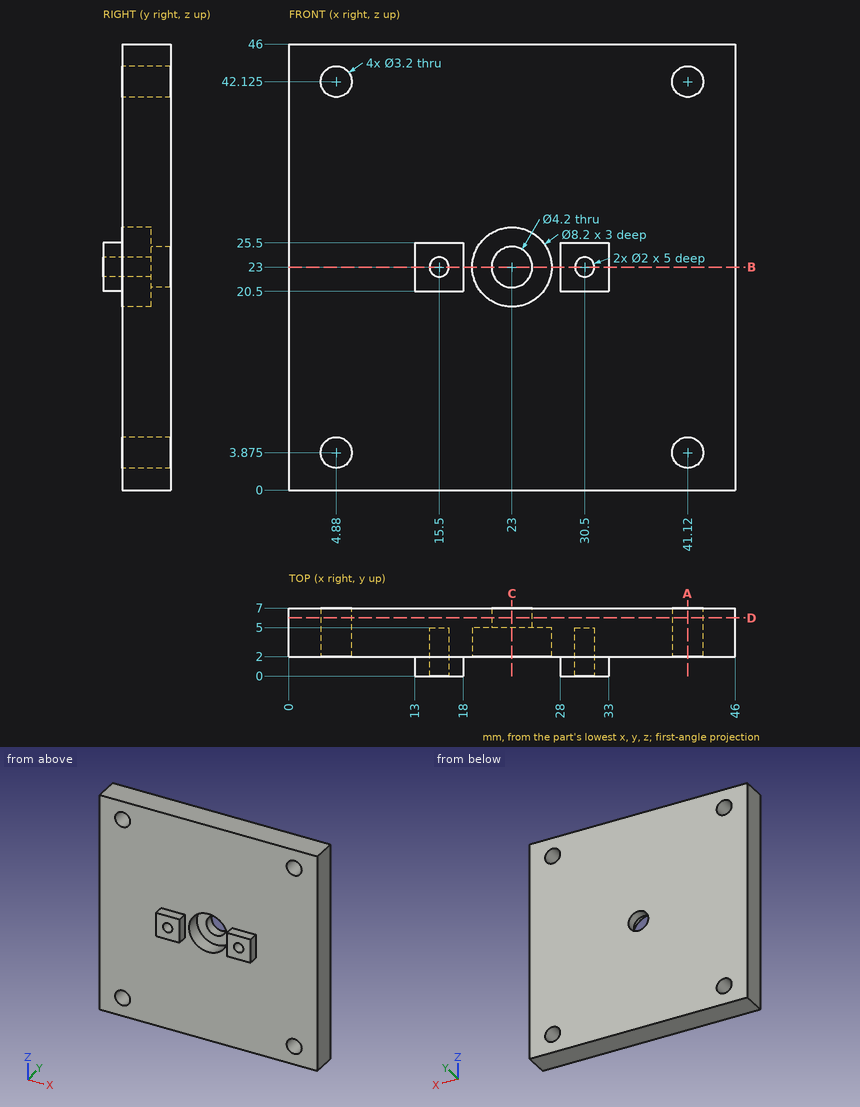
Here's the drawing with two shaded views (mm, measured from the low corner). I have some questions. Round coordinates to 2 decimals unless told otherwise and drop trailing zeros. Loops run counter-clockwise (first coordinate to the right, second up) from the corner with the lowest first, then second, coordinate; pieces in that order, holes last.
1. Suppose I cut it at A-A, the plane x = 41.12. Please give me the cut outline in (y, z) (3 decimals).
Answers:
outline: (2, 0) - (7, 0) - (7, 2.275) - (2, 2.275) - close; (2, 5.475) - (7, 5.475) - (7, 40.525) - (2, 40.525) - close; (2, 43.725) - (7, 43.725) - (7, 46) - (2, 46) - close
2. Suppose I cut it at B-B, the plane z = 23. Please give me the cut outline in (x, y), and give its area (3 significant figures).
Answers:
outline: (0, 2) - (13, 2) - (13, 0) - (14.5, 0) - (14.5, 5) - (16.5, 5) - (16.5, 0) - (18, 0) - (18, 2) - (18.9, 2) - (18.9, 5) - (20.9, 5) - (20.9, 7) - (0, 7) - close; (25.1, 5) - (27.1, 5) - (27.1, 2) - (28, 2) - (28, 0) - (29.5, 0) - (29.5, 5) - (31.5, 5) - (31.5, 0) - (33, 0) - (33, 2) - (46, 2) - (46, 7) - (25.1, 7) - close
area: 197 mm2
3. If I drill on probe 1 along X at (y, z) = (1.3, 23); probe 2 along Z at (x, y) = (23, 3.55); probe 3 along X at (y, z) = (4, 41), over which ranges is the centre line in solid material (lowest first)?
Answers:
probe 1: x = 13 to 14.5, 16.5 to 18, 28 to 29.5, 31.5 to 33
probe 2: z = 0 to 18.9, 27.1 to 46
probe 3: x = 0 to 3.74, 6.02 to 39.98, 42.26 to 46
4. Suppose I cut it at C-C, the plane x = 23. Please give me the cut outline in (y, z), and give its area (3 significant figures).
Answers:
outline: (2, 0) - (7, 0) - (7, 20.9) - (5, 20.9) - (5, 18.9) - (2, 18.9) - close; (2, 27.1) - (5, 27.1) - (5, 25.1) - (7, 25.1) - (7, 46) - (2, 46) - close
area: 197 mm2
5. Suppose I cut it at D-D, the plane y = 6. Please give me the cut outline in (x, z) (3 decimals).
Answers:
outline: (0, 0) - (46, 0) - (46, 46) - (0, 46) - close; hole circle Ø3.2 at (4.88, 3.875); hole circle Ø3.2 at (4.88, 42.125); hole circle Ø4.2 at (23, 23); hole circle Ø3.2 at (41.12, 3.875); hole circle Ø3.2 at (41.12, 42.125)
6. Will these pins go through, and if not, where does the flat tip stop? pin 1 (1.6 mm diameter, centred on y = 1, z = 23.5, fed in from +X); pin 2 (1.2 mm diameter, centred on x = 30.5, z = 23, fed in from -Y); pin 3 (6 mm diameter, centred on x = 35.5, z = 40.5, fed in from -Y).
Answers:
pin 1: stops at x = 33
pin 2: stops at y = 5
pin 3: stops at y = 2
